CAD build for the part. Positions are in the model's coordinates, mm. Face numbers are marked on the shaded views. Give positions to 0.01 mm unless a question says otherwise; leave off trailing zeros. Order: outer loops, then holes, each group sorted by start corner. A loop starts at its lowest first (then second) coordinate and runs counter-clockwise, first axis right, second up. Notation, with made-up numbers: (-20, -16.75) -> (6, -16.75) arc R11 cw to (6, -2.75) -> close; hole circle Ø6 at (27.25, 84.25). An arc over 180 degrees is marked (long way). Answer as CSV lines item,"result".
```python
from build123d import *

# Parameters (mm, degrees)
F0_R     = 16
F0_R_2   = 15
F1_DEPTH = 2
F2_DEPTH = 1
F3_R     = 1
F4_R     = 2


with BuildPart() as f1:
    # F0 (on Top) → F1 (new body)
    with BuildSketch(Plane.XY):
        Circle(F0_R)
        Circle(F0_R_2, mode=Mode.SUBTRACT)
        Circle(F0_R_2)
        Polygon((4.5, -4.5), (4.5, -12), (-4.5, -12), (-4.5, -4.5), (-12, -4.5), (-12, 4.5), (-4.5, 4.5), (-4.5, 12), (4.5, 12), (4.5, 4.5), (12, 4.5), (12, -4.5), align=None, mode=Mode.SUBTRACT)
    extrude(amount=F1_DEPTH)

    # F0 (on Top) → F2 (cut)
    with BuildSketch(Plane.XY):
        Circle(F0_R_2)
        Polygon((4.5, -4.5), (4.5, -12), (-4.5, -12), (-4.5, -4.5), (-12, -4.5), (-12, 4.5), (-4.5, 4.5), (-4.5, 12), (4.5, 12), (4.5, 4.5), (12, 4.5), (12, -4.5), align=None, mode=Mode.SUBTRACT)
    extrude(amount=F2_DEPTH, mode=Mode.SUBTRACT)

    # F3
    f3_edges = [f1.edges().sort_by_distance(p)[0] for p in [
        (-4.5, 12, 1.5),
        (4.5, 12, 1.5),
        (12, 4.5, 1.5),
        (12, -4.5, 1.5),
        (4.5, -12, 1.5),
        (-4.5, -12, 1.5),
        (-12, -4.5, 1.5),
        (-12, 4.5, 1.5),
    ]]
    fillet(f3_edges, radius=F3_R)

    # F4
    f4_edges = [f1.edges().sort_by_distance(p)[0] for p in [
        (-4.5, 4.5, 1.5),
        (4.5, 4.5, 1.5),
        (4.5, -4.5, 1.5),
        (-4.5, -4.5, 1.5),
    ]]
    fillet(f4_edges, radius=F4_R)


solid = f1.part
```
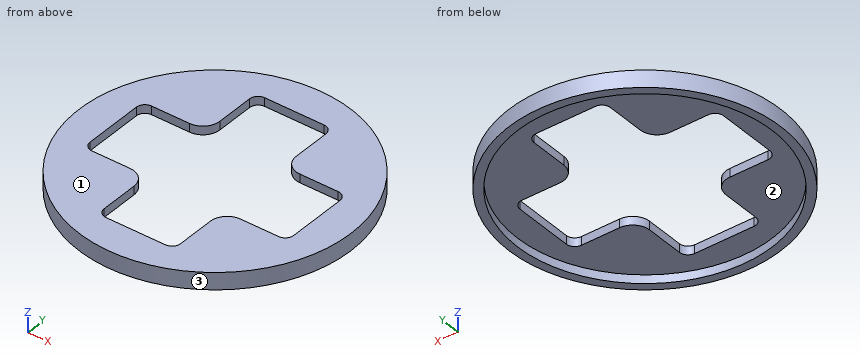
1) Wall check: line 1 along Y through (x, z) = (0, 0.8); line 2 along Z through (x, y) = (8, 10.5); line 3 along Y through (x, z) = (-11, 1.4). Give the ranges that are in metal, low to high. Write a range as [from, to].
Data:
line 1,"y = [-16, -15], [15, 16]"
line 2,"z = [1, 2]"
line 3,"y = [-11.62, -4.5], [4.5, 11.62]"
2) Band-saw the part on A-A, the plane x = 0. Write the cut outline in (y, z), then the cut area to 4 significant figures.
Data:
outline,"(-16, 0) -> (-15, 0) -> (-15, 1) -> (-12, 1) -> (-12, 2) -> (-16, 2) -> close; (12, 1) -> (15, 1) -> (15, 0) -> (16, 0) -> (16, 2) -> (12, 2) -> close"
area,"10.00 mm2"
3) Pull direction Y, two halves, no side cores. Call the marked faces 1, 2 and 3: pulls with the +Y half, pulls with the -Y half, needs draft (parallel to the pull), parting line crosses it, or undercut.
Data:
face 1,"needs draft"
face 2,"undercut"
face 3,"parting line crosses it"
4) Band-saw the part on C-C, the plane z = 1.45. Write the cut outline in (x, y).
Data:
outline,"circle Ø32 at (0, 0); hole (-12, -3.5) arc R1 ccw to (-11, -4.5) -> (-6.5, -4.5) arc R2 cw to (-4.5, -6.5) -> (-4.5, -11) arc R1 ccw to (-3.5, -12) -> (3.5, -12) arc R1 ccw to (4.5, -11) -> (4.5, -6.5) arc R2 cw to (6.5, -4.5) -> (11, -4.5) arc R1 ccw to (12, -3.5) -> (12, 3.5) arc R1 ccw to (11, 4.5) -> (6.5, 4.5) arc R2 cw to (4.5, 6.5) -> (4.5, 11) arc R1 ccw to (3.5, 12) -> (-3.5, 12) arc R1 ccw to (-4.5, 11) -> (-4.5, 6.5) arc R2 cw to (-6.5, 4.5) -> (-11, 4.5) arc R1 ccw to (-12, 3.5) -> close"
5) Band-saw the part on D-D, the plane x = -13. Write the cut outline in (y, z), then the cut area to 3 significant figures.
Data:
outline,"(-9.33, 0) -> (-7.48, 0) -> (-7.48, 1) -> (7.48, 1) -> (7.48, 0) -> (9.33, 0) -> (9.33, 2) -> (-9.33, 2) -> close"
area,"22.3 mm2"
6) Pin check, flat tips, straight feed: P1, Ø0.5, axis at y = 9.5, z = 1.5, coming from the -X side; P2, Ø0.8, axis at x = -9, z = 1.5, coming from the +Y side; P3, Ø1, axis at x = 0.5, y = -10.5, coming from the +Z side; P4, Ø0.5, axis at x = 8, z = 1.5, coming from the +Y side. Stop position of each tip, or through.
Data:
P1,"stops at x = -13.06"
P2,"stops at y = 13.49"
P3,"passes through"
P4,"stops at y = 14"
